Verification items for the finished model (mm, model axes). A direction names the side the tool comes from. Round coordinates to 2 decimals unless told otherwise and drop trailing zeros. Order: outer loops, then holes, each group sorted by start corner. A loop starts at its lowest first (then second) coordinate and runs counter-clockwise, first axis right, second up. Notation, with made-up numbers: M -2,-13 L 43,-13 A6 ccw 43,-6 Z; hole C 30.5,-7.75 d10. An arc over 180 degrees is marked long. Return JSON: item names as keys, results as strings. Group by question number.
from build123d import *

# Parameters (mm, degrees)
BOSS_EXTRUDE4_DEPTH = 13
BOSS_EXTRUDE5_DEPTH = 5
FILLET2_R           = 20
BOSS_EXTRUDE6_START = -42
SKETCH2_7_R         = 5
BOSS_EXTRUDE6_DEPTH = 42
SKETCH5_R           = 25
CUT_EXTRUDE1_DEPTH  = 42
SKETCH7_W           = 12
SKETCH7_H           = 10
CUT_EXTRUDE2_DEPTH  = 239
SKETCH8_R           = 5
CUT_EXTRUDE3_DEPTH  = 130
CUT_EXTRUDE4_DEPTH  = 130
CUT_EXTRUDE6_DEPTH  = 37


with BuildPart() as part:
    # Sketch2 → Boss-Extrude4 (new body)
    with BuildSketch(Plane(origin=(0, 0, 0), x_dir=(0, 0, -1), z_dir=(1, 0, 0))):
        with BuildLine():
            Line((0, 31.5), (0, 26.733616794))
            ThreePointArc((0, 26.733616794), (26.024128556, -6.118087921), (-11.911437782, -23.933322312))
            ThreePointArc((-11.911437782, -23.933322312), (-20.46059932, -28.4429224), (-30, -30))
            Line((-30, -30), (-30, -31.5))
            Line((-30, -31.5), (15, -31.5))
            Line((15, -31.5), (38.339650933, -23.005061782))
            ThreePointArc((38.339650933, -23.005061782), (43.924248506, -22.639027919), (48.830920178, -25.330920178))
            Line((48.830920178, -25.330920178), (55, -31.5))
            Line((55, -31.5), (70, -31.5))
            Line((70, -31.5), (70, -20))
            Line((70, -20), (50, -20))
            Line((50, -20), (50, 16.5))
            Line((50, 16.5), (30, 16.5))
            Line((30, 16.5), (30, 31.5))
            Line((30, 31.5), (0, 31.5))
        make_face()
        with BuildLine():
            ThreePointArc((5, 0), (3.535533906, 3.535533906), (0, 5))
            Line((0, 5), (0, 0))
            ThreePointArc((0, 0), (-0.104348142, -2.5), (-0.416666667, -4.982608643))
            ThreePointArc((-0.416666667, -4.982608643), (3.385016002, -3.679900361), (5, 0))
        make_face()
        with BuildLine():
            Line((0, 0), (0, 5))
            ThreePointArc((0, 5), (-3.549297202, 3.521716822), (-4.999847865, -0.03900425))
            ThreePointArc((-4.999847865, -0.03900425), (-3.666669267, -3.399343537), (-0.416666667, -4.982608643))
            ThreePointArc((-0.416666667, -4.982608643), (-0.104348142, -2.5), (0, 0))
        make_face()
        with BuildLine():
            ThreePointArc((-30, -30), (-20.46059932, -28.4429224), (-11.911437782, -23.933322312))
            ThreePointArc((-11.911437782, -23.933322312), (-15.61180413, -21.701563048), (-18.904262251, -18.902781162))
            ThreePointArc((-18.904262251, -18.902781162), (-24.302172741, -20.842036984), (-30, -21.5))
            Line((-30, -21.5), (-30, -30))
        make_face()
    extrude(amount=BOSS_EXTRUDE4_DEPTH)

    # Sketch2<6> → Boss-Extrude5 (add)
    with BuildSketch(Plane(origin=(0, 0, 0), x_dir=(0, 0, -1), z_dir=(1, 0, 0))):
        with BuildLine():
            ThreePointArc((-1.666666667, -9.860132972), (9.964971895, -0.836262603), (0, 10))
            Line((0, 10), (0, 5))
            ThreePointArc((0, 5), (3.535533906, 3.535533906), (5, 0))
            ThreePointArc((5, 0), (3.385016002, -3.679900361), (-0.416666667, -4.982608643))
            ThreePointArc((-0.416666667, -4.982608643), (-0.939156407, -7.447641886), (-1.666666667, -9.860132972))
        make_face()
    extrude(amount=BOSS_EXTRUDE5_DEPTH)

    # Fillet2
    fillet2_edges = [part.edges().sort_by_distance(p)[0] for p in [
        (6.5, -20, -50),
    ]]
    fillet(fillet2_edges, radius=FILLET2_R - 0.0001)  # a hair under: the kernel refuses the full size

    # Sketch2<7> → Boss-Extrude6 (add)
    with BuildSketch(Plane(origin=(0, 0, 0), x_dir=(0, 0, -1), z_dir=(1, 0, 0)).offset(BOSS_EXTRUDE6_START)):
        with BuildLine():
            Line((-30, -30), (-30, -31.5))
            Line((-30, -31.5), (15, -31.5))
            Line((15, -31.5), (38.339650933, -23.005061782))
            ThreePointArc((38.339650933, -23.005061782), (43.924248506, -22.639027919), (48.830920178, -25.330920178))
            Line((48.830920178, -25.330920178), (55, -31.5))
            Line((55, -31.5), (70, -31.5))
            Line((70, -31.5), (70, 16.5))
            Line((70, 16.5), (30, 16.5))
            Line((30, 16.5), (30, 31.5))
            Line((30, 31.5), (0, 31.5))
            Line((0, 31.5), (0, 0))
            ThreePointArc((0, 0), (-8.786796564, -21.213203436), (-30, -30))
        make_face()
        with Locations((60, 0)):
            Circle(SKETCH2_7_R, mode=Mode.SUBTRACT)
    extrude(amount=BOSS_EXTRUDE6_DEPTH)

    # Sketch5 → Cut-Extrude1 (cut)
    with BuildSketch(Plane(origin=(13, 0, 0), x_dir=(0, 0, -1), z_dir=(1, 0, 0))):
        with Locations((-30, 0)):
            Circle(SKETCH5_R)
    extrude(amount=-CUT_EXTRUDE1_DEPTH, mode=Mode.SUBTRACT)

    # Sketch7 → Cut-Extrude2 (cut)
    with BuildSketch(Plane(origin=(0, 31.5, 0), x_dir=(1, 0, 0), z_dir=(0, 1, 0))):
        with Locations((-36, 25)):
            Rectangle(SKETCH7_W, SKETCH7_H)
    extrude(amount=-CUT_EXTRUDE2_DEPTH, mode=Mode.SUBTRACT)

    # Sketch8 → Cut-Extrude3 (cut)
    with BuildSketch(Plane(origin=(0, 31.5, 0), x_dir=(1, 0, 0), z_dir=(0, 1, 0))):
        with Locations(Location((-17, 9, 0), (0, 0, 270))):
            Circle(SKETCH8_R)
    extrude(amount=-CUT_EXTRUDE3_DEPTH, mode=Mode.SUBTRACT)

    # Sketch9 → Cut-Extrude4 (cut)
    with BuildSketch(Plane.XY):
        Polygon((-42, 31.5), (-42, 13.5), (-35.448535783, 31.5), align=None)
    extrude(amount=-CUT_EXTRUDE4_DEPTH, mode=Mode.SUBTRACT)

    # Sketch10 → Cut-Extrude6 (cut)
    with BuildSketch(Plane.ZY.offset(42)):
        Polygon((-0.667060513, 13.5), (-20, 13.5), (-20, -29.680148829), (-15, -31.5), (-0.667060513, -31.5), align=None)
    extrude(amount=-CUT_EXTRUDE6_DEPTH, mode=Mode.SUBTRACT)


solid = part.part
1. Go/stop test with flat-tipped pins: pin 1 (22 mm diameter, centred on y = 4, z = -59.5, fed in from +X); pin 2 (5 mm diameter, centred on x = -31, y = -8.5, fed in from +Z); pin 3 (15.5 mm diameter, centred on y = -12.5, z = -10.5, fed in from -X); pin 4 (2 mm diameter, centred on x = -13, y = -12.5, fed in from +Z). Record where each tip stops, or that it passes through.
2. Cross-section at C-C (y = -8). Enter the section's corners in (x, z).
3. Access from +Z, -Z, +X, -X, +Y, -Y to the whole of each face (thin tool, end or side, straight path). Record for faces 1 (the face through (-8.77, -26.37, -29.1)), 2 (the face through (-24, 13.5, -10)), 3 (the face through (0, 0, 2)), 4 (the face through (-9, 24, -30)).
4. Cross-section at D-D (z = -25). Enter the section's corners in (x, y).
5. Thickness scan on line 1 along Z through (x, y) = (7.5, 0); line 2 along Z through (x, y) = (-33.5, 17.5); line 3 along X through (y, z) = (17.75, -9). Record the ranges inside material, lowest first. Write a range as from..to.
6. Cross-section at A-A (z = -59.5). Enter the section's corners in (x, y), plus the area to 3 significant figures.
7. Cross-section at B-B (y = 21). Enter the section's corners in (x, z), plus the area to 3 significant figures.
Computed:
{
 "1": {"pin 1": "stops at x = 13", "pin 2": "stops at z = 2.09", "pin 3": "stops at x = -5", "pin 4": "stops at z = 3.21"},
 "2": {"outline": "M -42,-70 L 0,-70 L 0,-51.67 L 13,-51.67 L 13,-25.51 L 0,-25.51 L 0,-6 L 5,-6 L 5,1.09 L -42,1.09 L -42,-0.67 L -5,-0.67 L -5,-20 L -30,-20 L -30,-30 L -42,-30 Z"},
 "3": {"face 1": "+X, -X, -Y", "face 2": "-X, -Y", "face 3": "+Z, -X, +Y", "face 4": "-Z, +X, -X, +Y"},
 "4": {"outline": "M -30,-27.86 L 13,-27.86 L 13,-9.47 L 0,-9.47 L 0,9.47 L 13,9.47 L 13,31.5 L -30,31.5 Z"},
 "5": {"line 1": "z = -50..-26.73, -5..5", "line 2": "z = -20..0", "line 3": "x = -40.45..-22, -12..0"},
 "6": {"outline": "M -42,-31.5 L 13,-31.5 L 13,-17.02 L 0,-17.02 L 0,-4.97 L -42,-4.97 Z; M -42,4.97 L 0,4.97 L 0,16.5 L -40.91,16.5 L -42,13.5 Z", "area": "1,780 mm²"},
 "7": {"outline": "M -39.27,-20 L -30,-20 L -30,-30 L 13,-30 L 13,-16.54 L 0,-16.54 L 0,0 L -39.27,0 Z; hole C -17,-9 d10", "area": "1,180 mm²"}
}
